Input: part model. Units: mm. Frame: model coordinates. A direction names the side the tool comes from. Round coordinates to 2 decimals unless told otherwise and drop trailing zeros. Loops run counter-clockwise (first coordinate to the right, second up) from the corner with the lowest first, then second, coordinate; pieces in that order, holes last. Notation, with made-up numbers: (70, -30) - (125, -30) arc R27 cw to (125, 6) - close; hole circle Ø3 at (72.5, 58.25). An arc over 180 degrees is marked (long way). One line per question, with ' | ' between items. Start each with the question number.
from build123d import *

# Parameters (mm, degrees)
EXTRUDE_1_DEPTH     = 9
SKETCH_3_R          = 11
CUT_EXTRUDE_1_DEPTH = 6
SKETCH_4_R          = 10
CUT_EXTRUDE_2_DEPTH = 4


with BuildPart() as part:
    # 스케치2 → 보스-돌출1 (new body)
    with BuildSketch(Plane(origin=(0, 0, 0), x_dir=(1, 0, 0), z_dir=(0, 1, 0))):
        with BuildLine():
            Line((-15, 0), (-15, -300))
            ThreePointArc((-15, -300), (0, -315), (15, -300))
            Line((15, -300), (15, 0))
            ThreePointArc((15, 0), (0, 15), (-15, 0))
        make_face()
    extrude(amount=EXTRUDE_1_DEPTH)

    # 스케치3 → 컷-돌출1 (cut)
    with BuildSketch(Plane(origin=(0, 9, 0), x_dir=(1, 0, 0), z_dir=(0, 1, 0))):
        Circle(SKETCH_3_R)
    extrude(amount=-CUT_EXTRUDE_1_DEPTH, mode=Mode.SUBTRACT)

    # 스케치4 → 컷-돌출2 (cut, through all)
    with BuildSketch(Plane(origin=(0, 3, 0), x_dir=(1, 0, 0), z_dir=(0, 1, 0))):
        Circle(SKETCH_4_R)
    extrude(amount=-CUT_EXTRUDE_2_DEPTH, mode=Mode.SUBTRACT)


solid = part.part
(1) Line query: line 1 along X through (y, z) = (7.8, 0); line 2 along Z through (x, y) = (0, 5.6); line 3 along Z through (x, y) = (-6.5, 6). Output: solid intervals per line, ascending. Write a range as from..to.
(2) Section A-A, the plane x = 0. Output: boundary loops of the cut face in (y, z).
(3) Pull-direction query (X, two-part tool) for faces 3 (the face through (-2.17, 1.52, 9.76)), 4 (the face through (2, 3, 10)), 5 (the face through (0, 4, -15)), 6 (the face through (15, 4, 152)); classes: released by +X, released by -X, zero draft, split by the parting line, or undercut.
(4) Reachability of faces 1 (the face through (0, 0, 148)), 2 (the face through (-2.38, 6.04, 10.74)) from +Z, -Z, +X, -X, +Y, -Y: full face, straight path, thin tool, end or side. Return the list, or none.
(5) Pin query (flat end, axial travel): P1, Ø18, axis at x = 0, z = 0, coming from the -Y side. Return the tip coordinate at first contact, or that it passes through.
(6) Section B-B, the plane y = 7. Output: boundary loops of the cut face in (x, z).
Derived:
1) line 1: x = -15..-11, 11..15 | line 2: z = -15..-11, 11..315 | line 3: z = -13.52..-8.87, 8.87..313.52
2) outline: (0, -15) - (9, -15) - (9, -11) - (3, -11) - (3, -10) - (0, -10) - close; (0, 10) - (3, 10) - (3, 11) - (9, 11) - (9, 315) - (0, 315) - close
3) face 3: undercut | face 4: undercut | face 5: split by the parting line | face 6: released by +X
4) face 1: +Z, -Z, +X, -X, -Y | face 2: +Y
5) P1: passes through
6) outline: (-15, 0) arc R15 ccw to (15, 0) - (15, 300) arc R15 ccw to (-15, 300) - close; hole circle Ø22 at (0, 0)
